Check sheet for the modelled part. Datum: model origin and axes. Units: mm. A direction names the side the tool comes from. Round coordinates to 2 decimals unless told otherwise and drop trailing zeros. Write each loop counter-clockwise with the first axis right and the second up, starting at its lowest first coordinate (ties: lowest second). Pieces come first, ordered by that corner, then holes. Notation, with made-up numbers: M 34,-17.5 L 80,-17.5 A21 ccw 80,15.5 Z; hole C 56,6.25 d1. An arc over 180 degrees is marked long. One line per item, written item: value.
Autodesk Inventor part; units mm, degrees
ref_plane "YZ Plane" through (0, 0, 0) normal (1, 0, 0) x (0, 1, 0)
ref_plane "XZ Plane" through (0, 0, 0) normal (0, 1, 0) x (-1, 0, 0)
ref_plane "XY Plane" through (0, 0, 0) normal (0, 0, 1) x (1, 0, 0)
sketch "Sketch1" plane through (0, 0, 0) normal (0, 1, 0) x (-1, 0, 0)
  circle A0 centre (0, 0) radius 7.5
  dimension "d0" = 15
extrude "Extrusion1" add sketch "Sketch1" along normal blind 30
chamfer "Chamfer1" distance 2 angle 45 1 edges at (7.5, 0, 0)
sketch "Sketch2" plane through (0, 30, 0) normal (0, 1, 0) x (1, 0, 0)
  circle A0 centre (0, 0) radius 12.5
  dimension "d6" = 25
extrude "Extrusion2" add sketch "Sketch2" along normal blind 5
chamfer "Chamfer2" distance 2 angle 45 1 edges at (-12.5, 35, 0)
thread "Thread1"
sketch "Sketch3" plane through (0, 35, 0) normal (0, 1, 0) x (1, 0, 0)
  circle A0 centre (0, 0) radius 5.5
  line L0 (0, 5.7735) -> (5, 2.8868)
  line L1 (5, 2.8868) -> (5, -2.8868)
  line L2 (5, -2.8868) -> (0, -5.7735)
  line L3 (0, -5.7735) -> (-5, -2.8868)
  line L4 (-5, -2.8868) -> (-5, 2.8868)
  line L5 (-5, 2.8868) -> (0, 5.7735)
  dimension "d14" = 10
extrude "Extrusion3" cut sketch "Sketch3" against normal blind 5 contours L1 A0 L2 L3 L4 L5 L0 | A0 L0 L1 | L1 L2 A0 | A0 L5 L0 | L2 L3 A0 | A0 L4 L5 | L3 L4 A0
properties part number "Tutorial_001_Bolt" material "Stainless Steel"
Q1. Draft check along Z on faces 4 (the conical face through (1.219, 0.125, -5.491)), 5 (the flat face through (-5, 33, 0)), 6 (the flat face through (2, 35, 5)). Enter one of: pulls with the +Z half, pulls with the -Z half, needs draft (parallel to the pull), parting line crosses it, or undercut.
Completed:
face 4: parting line crosses it
face 5: undercut
face 6: needs draft
Q2. Sectioned sample at B-B on y = 31. Enter the section's corners in (x, z), and give its area (3 significant figures).
Completed:
outline: C 0,0 d25; hole M -5,-2.89 L 0,-5.77 L 5,-2.89 L 5,2.89 L 0,5.77 L -5,2.89 Z
area: 404 mm^2
Q3. Sectioned sample at A-A on z = 0. Enter the section's corners in (x, y).
Completed:
outline: M -12.5,30 L -7.5,30 L -7.5,2 L -5.5,0 L 5.5,0 L 7.5,2 L 7.5,30 L 12.5,30 L 12.5,33 L 10.5,35 L 5,35 L 5,30 L -5,30 L -5,35 L -10.5,35 L -12.5,33 Z
Q4. Scan lines: line 1 (X direction, y = 31.5, z = 0.25); line 2 (Y direction, x = 5.5, z = 8.25); line 3 (Y direction, x = 1.5, z = -3.5). Record each from-to range of solid material in increasing order. Write a range as [from, to].
Completed:
line 1: [-12.5, -5], [5, 12.5]
line 2: [30, 35]
line 3: [0, 30]
Q5. Access from +Z, -Z, +X, -X, +Y, -Y to the whole of each face (thin tool, end or side, straight path). Record for faces 1 (the flat face through (0, 0, 0)), 2 (the flat face through (2.535, 32.535, 4.31)), 3 (the cylindrical face through (7.493, 15.804, -0.33)).
Completed:
face 1: +Z, -Z, +X, -X, -Y
face 2: +Y
face 3: -Y
Q6. Depth check by flat-ended pin: P1, Ø3, axis at x = -5, y = 13.5, coming from the -Z side; P2, Ø3, axis at y = 7, z = -7.5, coming from the +X side; P3, Ø2, axis at x = 4, z = 9, coming from the -Y side. Enter the tip coordinate at first touch or a pass-through.
Completed:
P1: z = -6.63
P2: x = 4.5
P3: y = 30
Q7. Sectioned sample at C-C on y = 7. Enter the section's corners in (x, z), and give its area (3 significant figures).
Completed:
outline: C 0,0 d15
area: 177 mm^2
